For this review, use the dimensioned drawing (mm, ordinates from the lowest corner) and the shaded views. A direction names the side the tool comes from. Coordinates: 2 decimals unless noted, no trailing zeros. Loops run counter-clockwise (first coordinate to the right, second up) from the corner with the lowest first, then second, coordinate; pieces in that order, holes last. Notation, with made-up numbers: M 50,-15 L 73,-15 A20 cw 73,22 Z; hole C -40,75 d2. An arc over 180 degrees is marked long. Write each question's results on one line, items separated by ' | '. Start each with the question number.
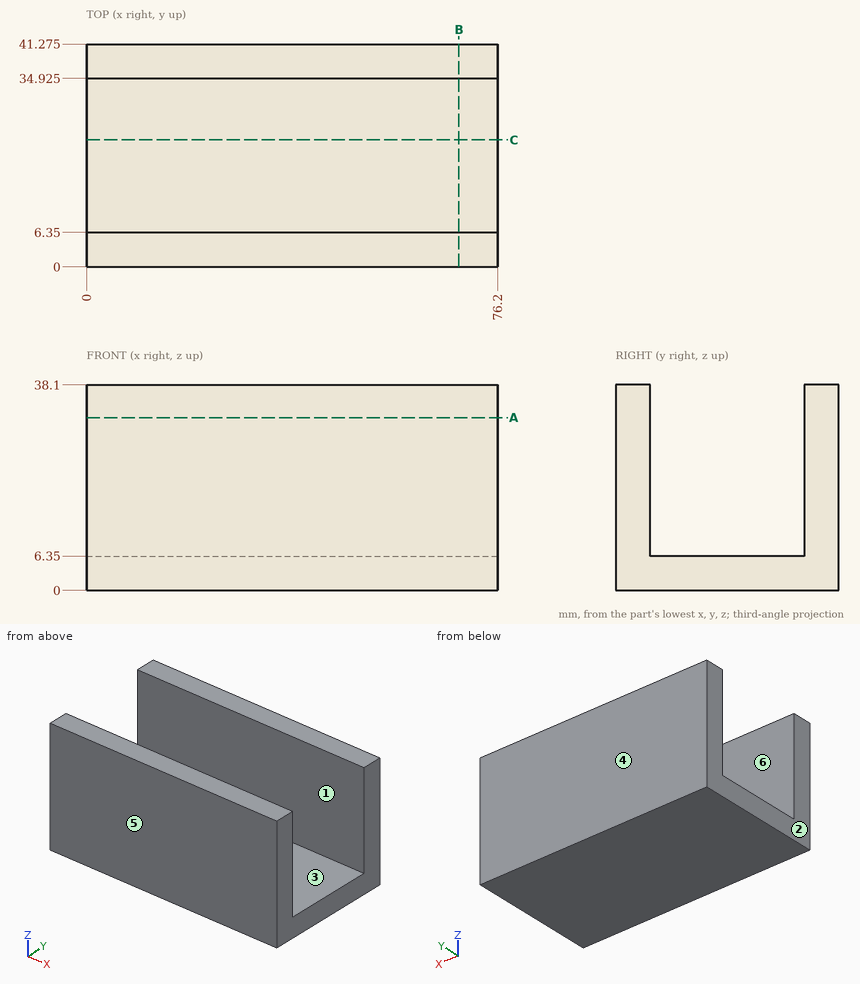
Q1. For the marked faces 5 and 6, list the 3-axis set-ups (+Z, -Z, +X, -X, +Y, -Y) from which the entire face can be reached by the end or side of a thin tool; tool diameter is ignored.
Q2. Take a section at A-A, the plane z = 32. Give the boundary of the cut face in (x, y) (3 decimals), then the cut area to 3 significant figures.
Q3. Take a section at C-C, the plane y = 23.5. Give the boundary of the cut face in (x, z), then the cut area to 3 significant figures.
Q4. Take a section at B-B, the plane x = 69. Give the boundary of the cut face in (y, z) (3 decimals), then the cut area to 3 significant figures.
Q5. To check wall thickness, follow line 1 along Y through (x, z) = (34, 12.5) (3 decimals); line 2 along Z through (x, y) = (21, 22). State the ranges of each line that lie inside material, in increasing order.
Q6. Insertion check: P1, Ø8.5, axis at x = 29, y = 26, coming from the +Z side; P2, Ø1.5, axis at x = 14.5, z = 32.5, coming from the -Y side. Each pin has a flat end and moves straight along its axis. Give the tip position at first contact, or say it passes through.
Q7. The part is to be moulded in two halves that separate along Y. For the marked faces 1, 2, 3 and 4, say which applies: pulls with the +Y half, pulls with the -Y half, needs draft (parallel to the pull), parting line crosses it, or undercut.
Results:
1) face 5: +Z, -Z, +X, -X, -Y | face 6: +Z, +X, -X
2) outline: M 0,0 L 76.2,0 L 76.2,6.35 L 0,6.35 Z; M 0,34.925 L 76.2,34.925 L 76.2,41.275 L 0,41.275 Z | area: 968 mm^2
3) outline: M 0,0 L 76.2,0 L 76.2,6.35 L 0,6.35 Z | area: 484 mm^2
4) outline: M 0,0 L 41.275,0 L 41.275,38.1 L 34.925,38.1 L 34.925,6.35 L 6.35,6.35 L 6.35,38.1 L 0,38.1 Z | area: 665 mm^2
5) line 1: 0 to 6.35, 34.925 to 41.275 | line 2: 0 to 6.35
6) P1: z = 6.35 | P2: y = 0
7) face 1: undercut | face 2: needs draft | face 3: undercut | face 4: pulls with the +Y half
